Input: dimensioned drawing with shaded views. Units: mm. Origin: part minimum x, y, z. Coordinates: 2 decimals unless noted, no trailing zeros. Order: outer loops, then holes, each group sorted by start corner. A loop starts at its lowest first (then second) coordinate and runs counter-clockwise, first axis right, second up. Notation, with made-up numbers: (27, 80) -> (45, 80) arc R32 ccw to (45, 118) -> close; hole circle Ø5 at (57.5, 59). An arc over 180 degrees is marked (long way). Answer in a Markdown table with one row per item. Add a question column.
1) Section query B-B on y = 8.5. Return the cut outline in (x, z) (1 decimal), then the cut area to 3 significant figures.
2) Section query A-A on x = 13.5. Return the cut outline in (y, z), then the cut area to 3 significant figures.
3) Contact query for flat-ended pins moving along their axis: P1, Ø6, axis at y = 6, z = 20, coming from the -X side; P2, Ø5, axis at x = 8.89, z = 20.32, coming from the +Y side; P3, Ø2, axis at y = 4.5, z = 26, coming from the -X side. Output: stop coordinate, or through.
4) Pull-direction query (Z, two-part tool) for the marked faces 1, 2 and 3; classes: +Z half, -Z half, draft (parallel to the pull), parting line (faces both ways), or undercut.
5) Ray query, line 1 (Y direction, x = 15, z = 39.5); line 2 (X direction, y = 10.2, z = 20.32) (1 decimal); line 3 (Z direction, x = 20.5, y = 4.5). Return the intervals inside material, ascending. Write a range as from..to.
6) Section query C-C on z = 13.5. Return the cut outline in (x, y).
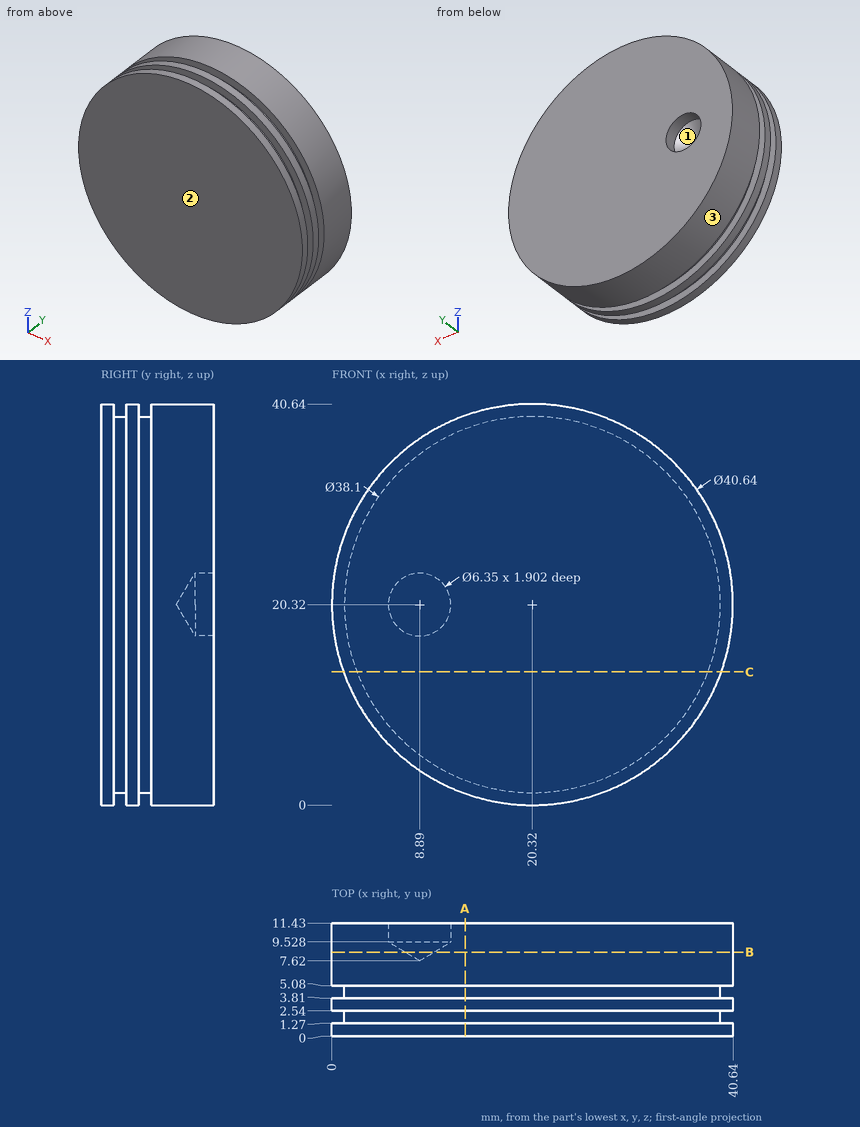
Result:
| question | item | result |
|---|---|---|
| 1 | outline | circle Ø40.6 at (20.3, 20.3); hole circle Ø2.9 at (8.9, 20.3) |
| 1 | area | 1,290 mm2 |
| 2 | outline | (0, 1.18) -> (1.27, 1.18) -> (1.27, 2.53) -> (2.54, 2.53) -> (2.54, 1.18) -> (3.81, 1.18) -> (3.81, 2.53) -> (5.08, 2.53) -> (5.08, 1.18) -> (11.43, 1.18) -> (11.43, 39.46) -> (5.08, 39.46) -> (5.08, 38.11) -> (3.81, 38.11) -> (3.81, 39.46) -> (2.54, 39.46) -> (2.54, 38.11) -> (1.27, 38.11) -> (1.27, 39.46) -> (0, 39.46) -> close |
| 2 | area | 431 mm2 |
| 3 | P1 | x = 0 |
| 3 | P2 | y = 9.12 |
| 3 | P3 | x = 0.59 |
| 4 | face 1 | undercut |
| 4 | face 2 | draft |
| 4 | face 3 | parting line |
| 5 | line 1 | 0..1.27, 2.54..3.81, 5.08..11.43 |
| 5 | line 2 | 0..5.7, 12.1..40.6 |
| 5 | line 3 | 1.27..39.37 |
| 6 | outline | (1.18, 0) -> (39.46, 0) -> (39.46, 1.27) -> (38.11, 1.27) -> (38.11, 2.54) -> (39.46, 2.54) -> (39.46, 3.81) -> (38.11, 3.81) -> (38.11, 5.08) -> (39.46, 5.08) -> (39.46, 11.43) -> (1.18, 11.43) -> (1.18, 5.08) -> (2.53, 5.08) -> (2.53, 3.81) -> (1.18, 3.81) -> (1.18, 2.54) -> (2.53, 2.54) -> (2.53, 1.27) -> (1.18, 1.27) -> close |
